Can you work these out from the model? Positions are in its coordinate system, mm. A direction names the side the tool comes from. Coordinates: 2 decimals unless noted, no trailing zeros. Write each loop counter-clockwise with the first axis right and the second up, starting at its lowest first coordinate (ties: lowest second). Pieces come first, ordered by that corner, then holes. Notation, with made-up numbers: (5, -3) -> (17, -3) arc R15 cw to (17, 6) -> close; hole circle Ø2 at (50.25, 44.5). An arc over 180 degrees is marked (long way). Use one line per item in the form item = value.
```python
from build123d import *

# Parameters (mm, degrees)
BOSS_EXTRUDE1_DEPTH = 11
SKETCH2_R           = 5
BOSS_EXTRUDE2_DEPTH = 11
SKETCH3_R           = 3.25
BOSS_EXTRUDE3_DEPTH = 1
FILLET1_R           = 2
CUT_EXTRUDE1_DEPTH  = 0.1


with BuildPart() as part:
    # Sketch1 → Boss-Extrude1 (new, symmetric)
    with BuildSketch(Plane.XY):
        with BuildLine():
            Line((-49, -38.5), (49, -38.5))
            ThreePointArc((49, -38.5), (56.071067812, -35.571067812), (59, -28.5))
            Line((59, -28.5), (59, 28.5))
            ThreePointArc((59, 28.5), (56.071067812, 35.571067812), (49, 38.5))
            Line((49, 38.5), (-49, 38.5))
            ThreePointArc((-49, 38.5), (-56.071067812, 35.571067812), (-59, 28.5))
            Line((-59, 28.5), (-59, -28.5))
            ThreePointArc((-59, -28.5), (-56.071067812, -35.571067812), (-49, -38.5))
        make_face()
    extrude(amount=BOSS_EXTRUDE1_DEPTH, both=True)

    # Sketch2 → Boss-Extrude2 (add, symmetric)
    with BuildSketch(Plane(origin=(0, 38.5, 0), x_dir=(1, 0, 0), z_dir=(0, 1, 0))):
        with Locations(Location((-40, 0, 0), (0, 0, 90))):
            Circle(SKETCH2_R)
        with Locations(Location((40, 0, 0), (0, 0, 90))):
            Circle(SKETCH2_R)
    extrude(amount=BOSS_EXTRUDE2_DEPTH, both=True)

    # Sketch3 → Boss-Extrude3 (add, symmetric)
    with BuildSketch(Plane(origin=(0, 0, -11), x_dir=(-1, 0, 0), z_dir=(0, 0, -1))):
        with Locations((-48, 31)):
            Circle(SKETCH3_R)
        with Locations((-48, -31)):
            Circle(SKETCH3_R)
        with Locations((48, -31)):
            Circle(SKETCH3_R)
        with Locations((48, 31)):
            Circle(SKETCH3_R)
    extrude(amount=BOSS_EXTRUDE3_DEPTH, both=True)

    # Fillet1
    # the kernel refuses this fillet: 2 mm, written as the material it takes off along each edge
    with BuildSketch(Plane(origin=(48, 31, -12), x_dir=(-1, 0, 0), z_dir=(0, -1, 0))) as fillet1_piece_1:
        with BuildLine():
            CenterArc((1.517949192, -2), FILLET1_R, 30, 60)
            Line((1.517949192, 0), (1.517949192, 0.04))
            Line((1.517949192, 0.04), (3.25, 0.04))
            Line((3.25, 0.04), (3.29, 0))
            ThreePointArc((3.29, 0), (3.29, -0.5), (3.284641016, -0.98))
            Line((3.284641016, -0.98), (3.25, -1))
        make_face()
    revolve(axis=Axis((48, 31, -12), (0, 0, -1)), mode=Mode.SUBTRACT)
    with BuildSketch(Plane(origin=(48, -31, -12), x_dir=(-1, 0, 0), z_dir=(0, -1, 0))) as fillet1_piece_2:
        with BuildLine():
            CenterArc((1.517949192, -2), FILLET1_R, 30, 60)
            Line((1.517949192, 0), (1.517949192, 0.04))
            Line((1.517949192, 0.04), (3.25, 0.04))
            Line((3.25, 0.04), (3.29, 0))
            ThreePointArc((3.29, 0), (3.29, -0.5), (3.284641016, -0.98))
            Line((3.284641016, -0.98), (3.25, -1))
        make_face()
    revolve(axis=Axis((48, -31, -12), (0, 0, -1)), mode=Mode.SUBTRACT)
    with BuildSketch(Plane(origin=(-48, -31, -12), x_dir=(-1, 0, 0), z_dir=(0, -1, 0))) as fillet1_piece_3:
        with BuildLine():
            CenterArc((1.517949192, -2), FILLET1_R, 30, 60)
            Line((1.517949192, 0), (1.517949192, 0.04))
            Line((1.517949192, 0.04), (3.25, 0.04))
            Line((3.25, 0.04), (3.29, 0))
            ThreePointArc((3.29, 0), (3.29, -0.5), (3.284641016, -0.98))
            Line((3.284641016, -0.98), (3.25, -1))
        make_face()
    revolve(axis=Axis((-48, -31, -12), (0, 0, -1)), mode=Mode.SUBTRACT)
    with BuildSketch(Plane(origin=(-48, 31, -12), x_dir=(-1, 0, 0), z_dir=(0, -1, 0))) as fillet1_piece_4:
        with BuildLine():
            CenterArc((1.517949192, -2), FILLET1_R, 30, 60)
            Line((1.517949192, 0), (1.517949192, 0.04))
            Line((1.517949192, 0.04), (3.25, 0.04))
            Line((3.25, 0.04), (3.29, 0))
            ThreePointArc((3.29, 0), (3.29, -0.5), (3.284641016, -0.98))
            Line((3.284641016, -0.98), (3.25, -1))
        make_face()
    revolve(axis=Axis((-48, 31, -12), (0, 0, -1)), mode=Mode.SUBTRACT)

    # Sketch4 → Cut-Extrude1 (cut)
    with BuildSketch(Plane.XY.offset(11)):
        with BuildLine():
            Line((-40, -28.5), (40, -28.5))
            ThreePointArc((40, -28.5), (42.828427125, -27.328427125), (44, -24.5))
            Line((44, -24.5), (44, -17.5))
            ThreePointArc((44, -17.5), (42.828427125, -14.671572875), (40, -13.5))
            Line((40, -13.5), (-40, -13.5))
            ThreePointArc((-40, -13.5), (-42.828427125, -14.671572875), (-44, -17.5))
            Line((-44, -17.5), (-44, -24.5))
            ThreePointArc((-44, -24.5), (-42.828427125, -27.328427125), (-40, -28.5))
        make_face()
    extrude(amount=-CUT_EXTRUDE1_DEPTH, mode=Mode.SUBTRACT)


solid = part.part
```
Q1. Thinking about a two-plate mould opening in X: for faces 1 (the cylindrical face through (-56.15, -35.49, 0.15)), 2 (the flat face through (40, 49.5, 0)), 3 (the cylindrical face through (35.043, 44.077, 0.651)), which applies, released by +X, released by -X, zero draft, split by the parting line, or undercut?
Return value:
face_1 = released by -X
face_2 = zero draft
face_3 = undercut
Q2. If I drill on line 1 (Z direction, x = 19, y = 6); line 2 (Y direction, x = -39, z = -10.25); line 3 (Z direction, x = 49.5, y = 30.5), over which ranges is the centre line in solid material (lowest first)? Write a range as from..to.
Return value:
line_1 = -11..11
line_2 = -38.5..38.5
line_3 = -12..11
Q3. Will these pins go through, and if not, where does the flat tip stop? pin 1 (3 mm diameter, centred on x = 21.5, y = 38, fed in from -Z); pin 2 (5 mm diameter, centred on x = 9, y = -17, fed in from +Z); pin 3 (8 mm diameter, centred on x = 8, z = 1, fed in from +Y).
Return value:
pin_1 = -11
pin_2 = 10.9
pin_3 = 38.5
Q4. For faces 4 (the flat face through (48, -31, -12)), 5 (the flat face through (-1, -21, 10.9)), which set-ups out of +Z, -Z, +X, -X, +Y, -Y let a thin tool reach every point of the face, with its end or its side?
Return value:
face_4 = -Z, +X, -X, +Y, -Y
face_5 = +Z
Q5. Suppose I cut it at C-C (y = 6.5). Write out the boundary of the cut face in (x, z), then the cut area to 3 significant figures.
Return value:
outline = (-59, -11) -> (59, -11) -> (59, 11) -> (-59, 11) -> close
area = 2,600 mm2
Q6. Suppose I cut it at A-A (x = 30.5). Write out the boundary of the cut face in (y, z).
Return value:
outline = (-38.5, -11) -> (38.5, -11) -> (38.5, 11) -> (-13.5, 11) -> (-13.5, 10.9) -> (-28.5, 10.9) -> (-28.5, 11) -> (-38.5, 11) -> close
Q7. Suppose I cut it at D-D (z = 0). Write out the boundary of the cut face in (x, y), then the cut area to 3 significant figures.
Return value:
outline = (-59, -28.5) arc R10 ccw to (-49, -38.5) -> (49, -38.5) arc R10 ccw to (59, -28.5) -> (59, 28.5) arc R10 ccw to (49, 38.5) -> (45, 38.5) -> (45, 49.5) -> (35, 49.5) -> (35, 38.5) -> (-35, 38.5) -> (-35, 49.5) -> (-45, 49.5) -> (-45, 38.5) -> (-49, 38.5) arc R10 ccw to (-59, 28.5) -> close
area = 9,220 mm2
Q8. Suppose I cut it at B-B (z = 8.25). Write out the boundary of the cut face in (x, y).
Return value:
outline = (-59, -28.5) arc R10 ccw to (-49, -38.5) -> (49, -38.5) arc R10 ccw to (59, -28.5) -> (59, 28.5) arc R10 ccw to (49, 38.5) -> (-49, 38.5) arc R10 ccw to (-59, 28.5) -> close
